Geometry check sheet. Reference: drawing and pictorial views, mm from the part's lowest x, y, z. A direction names the side the tool comes from. Give positions to 0.01 mm unless a question says otherwise; leave off trailing zeros. Loops run counter-clockwise (first coordinate to the right, second up) from the corner with the lowest first, then second, coordinate; pieces in that order, holes last. Notation, with made-up numbers: M 58,89 L 87,89 A23 ccw 87,125 Z; hole C 0,20.25 d5. An arc over 180 degrees is marked long. Use CSV: the item, a comma, the result in double quotes.
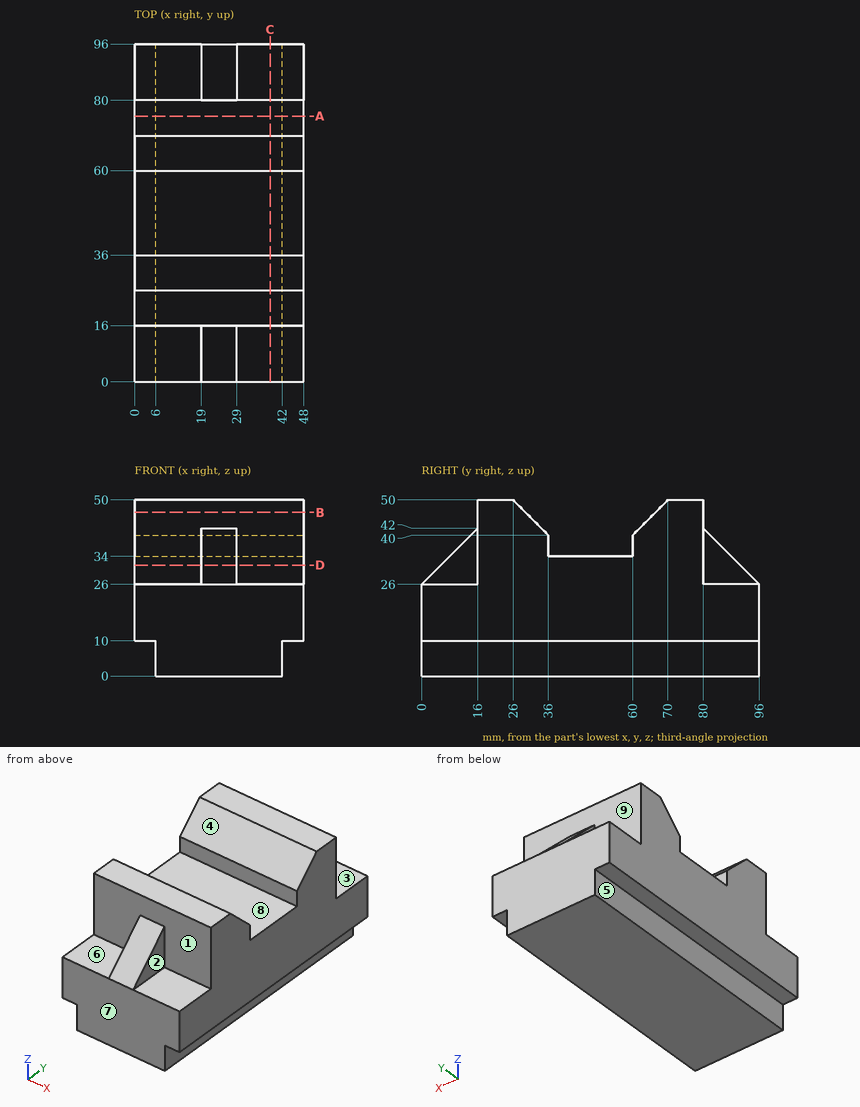
(1) Section check A-A on y = 75.5. Record the cut outline in (x, z).
Calculated:
outline,"M 0,10 L 6,10 L 6,0 L 42,0 L 42,10 L 48,10 L 48,50 L 0,50 Z"
(2) Tool access check on the marked faces 1, 2, 3, 4 and 5. Record the directions out of +Z, -Z, +X, -X, +Y, -Y that give a thin tool (end or side, any length) a straight path to the whole face; none if there is none.
Calculated:
face 1,"+Z, -Y"
face 2,"+Z, +X, -Y"
face 3,"+Z, +X, +Y"
face 4,"+Z, +X, -X"
face 5,"-Z, -X, +Y, -Y"
(3) Section check C-C on x = 38.5. Record the cut outline in (y, z), plus the area to 3 significant figures.
Calculated:
outline,"M 0,0 L 96,0 L 96,26 L 80,26 L 80,50 L 70,50 L 60,40 L 60,34 L 36,34 L 36,40 L 26,50 L 16,50 L 16,26 L 0,26 Z"
area,"3,550 mm²"
(4) Scan lines: L1, parallel to Y at x = 4, z = 37; L2, parallel to Z at x = 33, y = 52.5; L3, parallel to Y at x = 44.5, z = 32. Record each from-to range of solid material in increasing order. Write a range as from..to.
Calculated:
L1,"y = 16..36, 60..80"
L2,"z = 0..34"
L3,"y = 16..80"
(5) Section check D-D on z = 31.5. Record the cut outline in (x, y).
Calculated:
outline,"M 0,16 L 19,16 L 19,5.5 L 29,5.5 L 29,16 L 48,16 L 48,80 L 29,80 L 29,90.5 L 19,90.5 L 19,80 L 0,80 Z"
(6) Section check B-B on z = 46.5. Record the cut outline in (x, y), plus the area to 3 significant figures.
Calculated:
outline,"M 0,16 L 48,16 L 48,29.5 L 0,29.5 Z; M 0,66.5 L 48,66.5 L 48,80 L 0,80 Z"
area,"1,300 mm²"
(7) Mould release check, pull along Y, two halves, no side actions. Record for the marked faces 6, 7, 8 and 9: released by +Y, released by -Y, zero draft, split by the parting line, or undercut.
Calculated:
face 6,"zero draft"
face 7,"released by -Y"
face 8,"undercut"
face 9,"released by +Y"
(8) Depth check by flat-ended pin: pin 1 Ø1.5 at (x, y) = (38, 54.5) entering from +Z; pin 2 Ø1 at (x, z) = (28.5, 32) entering from -Y; pin 3 Ø10 at (x, z) = (8, 32) entering from +Y. Enter the tip coordinate at first touch or a pass-through.
Calculated:
pin 1,"stops at z = 34"
pin 2,"stops at y = 5.5"
pin 3,"stops at y = 80"
